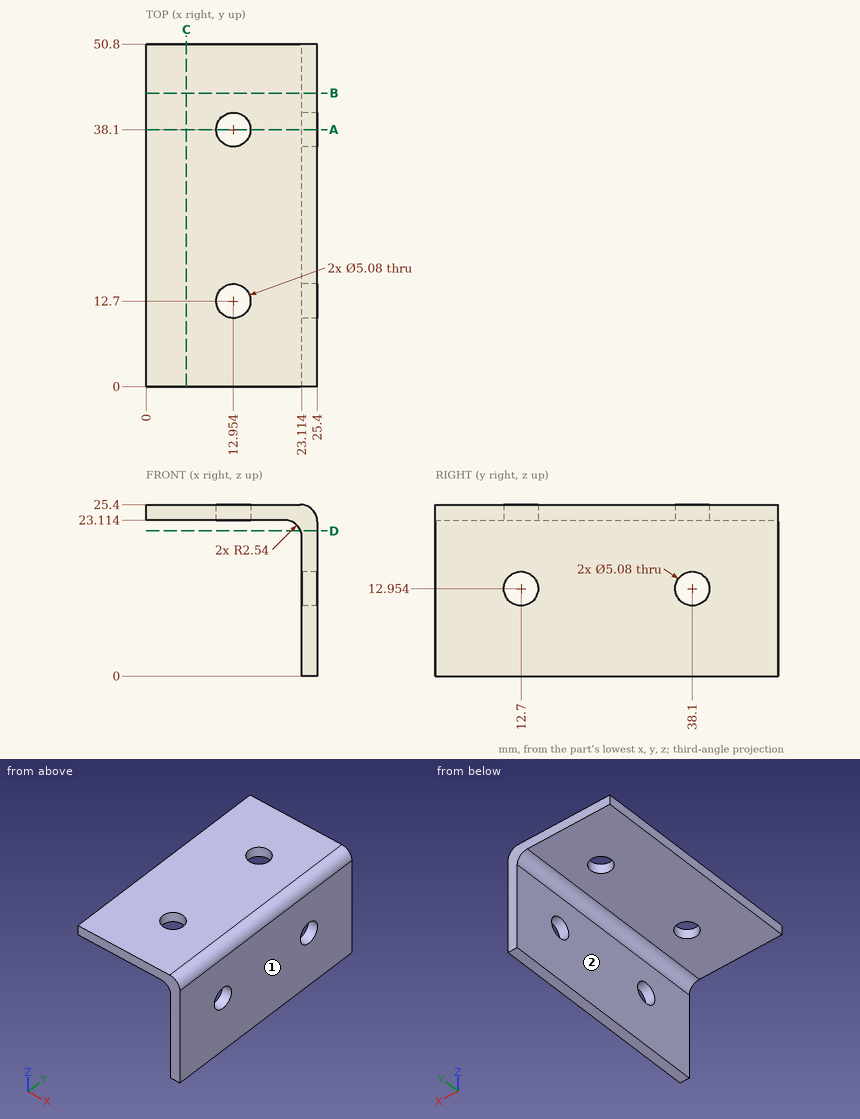
Geometry check sheet. Reference: drawing and pictorial views, mm from the part's lowest x, y, z. A direction names the side the tool comes from. Give positions to 0.01 mm unless a question says otherwise; leave off trailing zeros. Write each loop counter-clockwise with the first axis right and the second up, starting at its lowest first coordinate (ties: lowest second). Pieces come first, ordered by that corner, then holes. Notation, with made-up numbers: (-32.5, 40) - (14.5, 40) arc R11 cw to (14.5, 58) - close; hole circle Ø10 at (10.25, 18). An arc over 180 degrees is marked (long way). Use a Markdown table: item, result.
Q1. Set-up check for the marked faces 1 and 2: record each of +Z, -Z, +X, -X, +Y, -Y from which the full face is reachable in a straight line by a thin tool's end or side.
Computed:
| item | result |
|---|---|
| face 1 | +Z, -Z, +X, +Y, -Y |
| face 2 | -Z, -X, +Y, -Y |
Q2. Thickness scan on L1, parallel to Z at x = 16.25, y = 35; L2, parallel to Z at x = 21.25, y = 28. Record the ranges inside material, lowest first. Write a range as [from, to].
Computed:
| item | result |
|---|---|
| L1 | z = [23.11, 25.4] |
| L2 | z = [23.02, 25.4] |
Q3. Go/stop test with flat-tipped pins: P1, Ø2, axis at x = 10.5, y = 30, coming from the -Z side; P2, Ø8, axis at y = 38.1, z = 12.954, coming from the -X side; P3, Ø3, axis at x = 12.954, y = 38.1, coming from the +Z side. Record where each tip stops, or that it passes through.
Computed:
| item | result |
|---|---|
| P1 | stops at z = 23.11 |
| P2 | stops at x = 23.11 |
| P3 | passes through |
Q4. Section check C-C, the plane x = 6. Enter the section's corners in (y, z), then the cut area to 3 significant figures.
Computed:
| item | result |
|---|---|
| outline | (0, 23.11) - (50.8, 23.11) - (50.8, 25.4) - (0, 25.4) - close |
| area | 116 mm² |
Q5. Section check B-B, the plane y = 43.5. Enter the section's corners in (x, z), then the cut area to 3 significant figures.
Computed:
| item | result |
|---|---|
| outline | (0, 23.11) - (20.57, 23.11) arc R2.54 cw to (23.11, 20.57) - (23.11, 0) - (25.4, 0) - (25.4, 22.86) arc R2.54 ccw to (22.86, 25.4) - (0, 25.4) - close |
| area | 111 mm² |
Q6. Section check A-A, the plane y = 38.1. Enter the section's corners in (x, z).
Computed:
| item | result |
|---|---|
| outline | (0, 23.11) - (10.41, 23.11) - (10.41, 25.4) - (0, 25.4) - close; (15.49, 23.11) - (20.57, 23.11) arc R2.54 cw to (23.11, 20.57) - (23.11, 15.49) - (25.4, 15.49) - (25.4, 22.86) arc R2.54 ccw to (22.86, 25.4) - (15.49, 25.4) - close; (23.11, 0) - (25.4, 0) - (25.4, 10.41) - (23.11, 10.41) - close |
Q7. Section check D-D, the plane z = 21.5. Enter the section's corners in (x, y).
Computed:
| item | result |
|---|---|
| outline | (22.94, 0) - (25.4, 0) - (25.4, 50.8) - (22.94, 50.8) - close |
